```python
from build123d import *

# Parameters (mm, degrees)
F0_R     = 5.15
F0_R_2   = 13
F0_R_3   = 8.25
F1_DEPTH = 10
F3_R     = 13
F4_DEPTH = 30.041475


with BuildPart() as f1:
    # F0 (on Front) → F1 (new body)
    with BuildSketch(Plane.XZ):
        Polygon((115.000841, -20), (114.998738, 30), (-115.001262, 30), (-114.999159, -20), (-24.999159, -138), (25.000841, -138), align=None)
        with Locations((-35, -85)):
            Circle(F0_R, mode=Mode.SUBTRACT)
        with Locations((0, -106.326342)):
            Circle(F0_R_2, mode=Mode.SUBTRACT)
        with Locations((35, -85)):
            Circle(F0_R, mode=Mode.SUBTRACT)
        with Locations((-64.998738, 0)):
            Circle(F0_R_3, mode=Mode.SUBTRACT)
        with Locations((64.998738, 0)):
            Circle(F0_R_3, mode=Mode.SUBTRACT)
    extrude(amount=F1_DEPTH)

    # F3 (on face) → F4 (cut, through all)
    with BuildSketch(Plane(origin=(0, 15.543407, -2.322978), x_dir=(-1, 0, 0), z_dir=(0, 0.989016, -0.147809))):
        with Locations((0, -105.158439)):
            Circle(F3_R)
    extrude(amount=-F4_DEPTH, mode=Mode.SUBTRACT)


solid = f1.part
```
Read the model definition and answer for the solid it produces. Units are mm, in the model's axes. Give positions to 0.01 mm unless a question says otherwise; leave off trailing zeros. Order: outer loops, then holes, each group sorted by start corner. A loop starts at its lowest first (then second) coordinate and runs counter-clockwise, first axis right, second up. Notation, with made-up numbers: (-3.5, 29.5) -> (19.5, 29.5) arc R33 cw to (19.5, 64.5) -> close; hole circle Ø8 at (52.25, 2.5). An arc over 180 degrees is marked (long way). One line per item, written item: value. Start each with the question number.
(1) The part is cut by section B-B (x = 35). Determine the outline of the cut face in (y, z).
(2) The part is cut by section C-C (x = -9). Determine the outline of the cut face in (y, z).
(3) Flat-ended cylindrical pins translate along their axes: P1, Ø1.5, axis at y = -5, z = -94, coming from the -X side; P2, Ø15, axis at x = 65, z = 0, coming from the +Y side; P3, Ø1.5, axis at y = -6, z = -76, coming from the +X side; P4, Ø2, axis at y = -2.5, z = -95, coming from the +X side. Find the tip coordinate at first contact, or state that the pin passes through.
(4) The part is cut by section D-D (y = -6). State how many separate pieces and enclosed holes the cut face has, and give its area (3 significant figures).
(5) For a pull along Z with two mould halves and no side action, classify faces 1 (the flat face through (2, -5, 30)), 2 (the cylindrical face through (-0.296, -4.93, -119.323)), 3 (the cylindrical face through (33.884, -4.93, -90.028)), 4 (the flat face through (-2, -10, -34)) as released by +Z, released by -Z, zero draft, split by the parting line, or undercut.
(6) Straight lines are drawn through the part: L1, parallel to X at y = -5.75, z = -9; L2, parallel to Z at x = -12, y = -4.5; L3, parallel to Z at x = -70, y = -0.5. For each, find the intervals that lie inside material, in ascending order.
(7) The part is cut by section A-A (z = 0). Determine the outline of the cut face in (x, y), and give its area (3 significant figures).
Taken from the geometry:
1. outline: (-10, -124.89) -> (0, -124.89) -> (0, -90.15) -> (-10, -90.15) -> close; (-10, -79.85) -> (0, -79.85) -> (0, 30) -> (-10, 30) -> close
2. outline: (-10, -138) -> (0, -138) -> (0, -115.71) -> (-10, -115.71) -> close; (-10, -95.35) -> (0, -96.84) -> (0, 30) -> (-10, 30) -> close
3. P1: x = -59.13
3. P2: through
3. P3: x = 72.86
3. P4: x = 58.56
4. separate pieces: 1
4. enclosed holes: 5
4. area: 26,900 mm^2
5. face 1: released by +Z
5. face 2: undercut
5. face 3: undercut
5. face 4: zero draft
6. L1: -115 to 115
6. L2: -138 to -111.33, -100.6 to 30
6. L3: -79 to -6.56, 6.56 to 30
7. outline: (-115, -10) -> (-73.25, -10) -> (-73.25, 0) -> (-115, 0) -> close; (-56.75, -10) -> (56.75, -10) -> (56.75, 0) -> (-56.75, 0) -> close; (73.25, -10) -> (115, -10) -> (115, 0) -> (73.25, 0) -> close
7. area: 1,970 mm^2
